Check sheet for the drawn part. Datum: minimum x, y, z corner. Units: mm. A direction names the side the tool comes from. Give positions to 0.01 mm unless a question says otherwise; leave off trailing zeros. Write each loop counter-clockwise with the first axis right and the second up, starting at its lowest first coordinate (ties: lowest second). Pieces come first, ordered by that corner, then holes. Notation, with made-up numbers: M 79,61 L 128,61 A18 cw 128,72 Z; hole C -5,51.25 d10. An arc over 180 degrees is marked long. Write item = value, one per line.
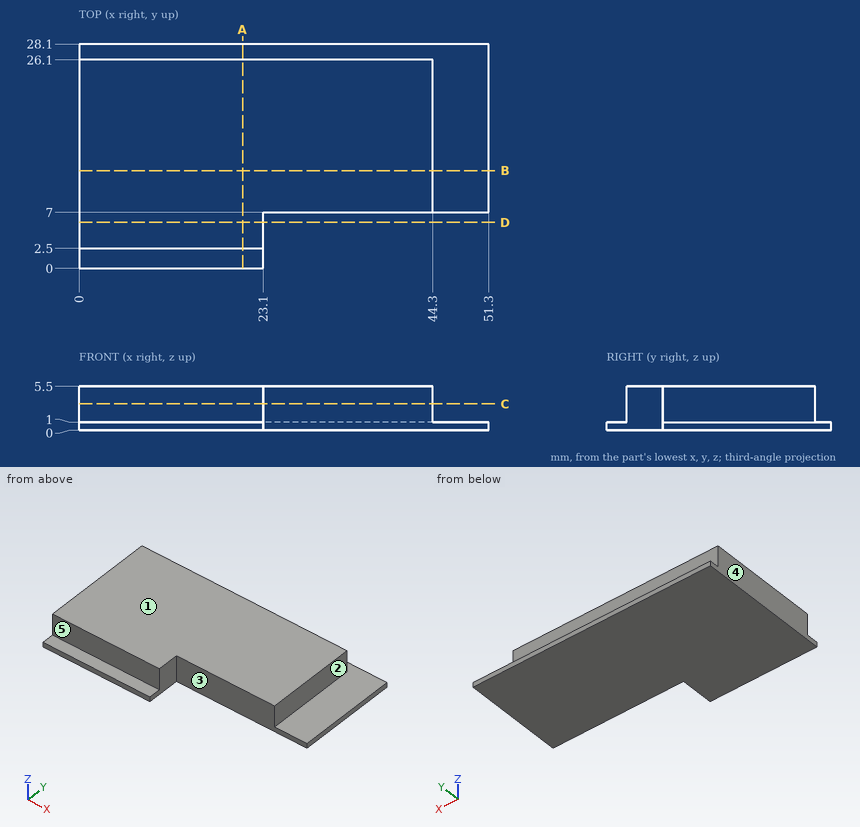
1) Material ranges on probe 1 along Y at (x, z) = (17.5, 3.2); probe 2 along Y at (x, z) = (25, 5.15); probe 3 along Z at (x, y) = (47, 21.5), recorded low to high. Write a range as from..to.
From the geometry:
probe_1 = 2.5..26.1
probe_2 = 7..26.1
probe_3 = 0..1
2) Cross-section at D-D on y = 5.75. Record the boundary of the cut face in (x, z), plus the area to 3 significant figures.
From the geometry:
outline = M 0,0 L 23.1,0 L 23.1,5.5 L 0,5.5 Z
area = 127 mm^2
3) Cross-section at C-C on z = 3.3. Record the boundary of the cut face in (x, y), plus the area to 3 significant figures.
From the geometry:
outline = M 0,2.5 L 23.1,2.5 L 23.1,7 L 44.3,7 L 44.3,26.1 L 0,26.1 Z
area = 950 mm^2
4) Depth check by flat-ended pin: P1, Ø0.8, axis at x = 12, y = 0.5, coming from the +Z side; P2, Ø1.3, axis at x = 22, z = 3.5, coming from the +Y side; P3, Ø3, axis at x = 21.5, z = 4, coming from the -Y side. Enter the tip coordinate at first touch or a pass-through.
From the geometry:
P1 = 1
P2 = 26.1
P3 = 2.5
5) Cross-section at A-A on x = 20.5. Record the boundary of the cut face in (y, z), plus the area to 3 significant figures.
From the geometry:
outline = M 0,0 L 28.1,0 L 28.1,1 L 26.1,1 L 26.1,5.5 L 2.5,5.5 L 2.5,1 L 0,1 Z
area = 134 mm^2
6) Cross-section at B-B on y = 12.25. Record the boundary of the cut face in (x, z), plus the area to 3 significant figures.
From the geometry:
outline = M 0,0 L 51.3,0 L 51.3,1 L 44.3,1 L 44.3,5.5 L 0,5.5 Z
area = 251 mm^2
7) Tool access check on the marked faces 1, 2, 3, 4 and 5. Record the directions out of +Z, -Z, +X, -X, +Y, -Y that give a thin tool (end or side, any length) a straight path to the whole face; none if there is none.
From the geometry:
face_1 = +Z, +X, -X, +Y, -Y
face_2 = +Z, +X, +Y, -Y
face_3 = +Z, -Z, +X, -Y
face_4 = +Z, -Z, -X, +Y, -Y
face_5 = +Z, +X, -X, -Y
